from build123d import *

# Parameters (mm, degrees)
F1_DEPTH = 9.8
F2_R     = 1.75
F3_DEPTH = 7
F4_R     = 1.75
F5_DEPTH = 7
F6_W     = 115
F6_H     = 2.2
F7_DEPTH = 7.5
F8_W     = 113.41
F8_H     = 1.6
F9_DEPTH = 233
F10_R    = 2


with BuildPart() as f1:
    # F0 (on Top) → F1 (new body)
    with BuildSketch(Plane.XY):
        Polygon((8.22, 6), (0, 6), (0, 0), (7, 0), (7, -4.8), (125.55, -4.8), (125.55, 0), (132.55, 0), (132.55, 6), (124.33, 6), (124.33, 10), (122.98, 10), (122.98, 6), (9.57, 6), (9.57, 10), (8.22, 10), align=None)
    extrude(amount=F1_DEPTH)

    # F2 (on face) → F3 (cut)
    with BuildSketch(Plane.XZ):
        with Locations((3.5, 4.9)):
            Circle(F2_R)
    extrude(amount=-F3_DEPTH, mode=Mode.SUBTRACT)

    # F4 (on face) → F5 (cut)
    with BuildSketch(Plane.XZ):
        with Locations((129.05, 4.9)):
            Circle(F4_R)
    extrude(amount=-F5_DEPTH, mode=Mode.SUBTRACT)

    # F6 (on face) → F7 (cut)
    with BuildSketch(Plane.XZ.offset(4.8)):
        with Locations((66.275, 4.9)):
            Rectangle(F6_W, F6_H)
    extrude(amount=-F7_DEPTH, mode=Mode.SUBTRACT)

    # F8 (on face) → F9 (join)
    with BuildSketch(Plane(origin=(0, 6, 0), x_dir=(-1, 0, 0), z_dir=(0, 1, 0))):
        with Locations((-66.275, 4.9)):
            Rectangle(F8_W, F8_H)
    extrude(amount=F9_DEPTH)

    # F10
    f10_edges = [f1.edges().sort_by_distance(p)[0] for p in [
        (122.98, 239, 4.9),
        (9.57, 239, 4.9),
    ]]
    fillet(f10_edges, radius=F10_R)


solid = f1.part
Model file for the job. Use its own axes, mm. A direction names the side the tool comes from. Give positions to 0.01 mm unless a question says otherwise; leave off trailing zeros. Loops run counter-clockwise (first coordinate to the right, second up) from the corner with the lowest first, then second, coordinate; pieces in that order, holes last.
1) Wall check: line 1 (Z direction, x = 3.5, y = 3.45); line 2 (Z direction, x = 69, y = 84.5); line 3 (Y direction, x = 124, z = 0.5). Give the ranges that are in metal, low to high.
2) Tool access for faces 4 (the flat face through (7, -2, 5)), 5 (the flat face through (127, 6, 5)), 6 (the flat face through (125.55, -2, 5)): list every direction of +Z, -Z, +X, -X, +Y, -Y with a clear straight run to the whole face (end or side of a thin tool).
3) Saw through at B-B (x = 72). Write the cut outline in (y, z).
4) Saw through at C-C (y = 118). Write the cut outline in (x, z).
5) Saw through at A-A (z = 1.5). Write the cut outline in (x, y).
6) Flat gauge pins, fed straight in: pin 1 Ø1.2 at (y, z) = (7, 2) entering from +X; pin 2 Ø3 at (y, z) = (8.5, 7.5) entering from -X; pin 3 Ø3 at (x, z) = (3.5, 4.9) entering from +Y; pin 4 Ø1 at (x, z) = (32, 2) entering from +Y. Where does each tip first touch, or does it go through?
7) Pull direction Z, two halves, no side cores. Call faces 1 (the flat face through (65, -1, 6)), 2 (the flat face through (132.55, 3, 5)), 3 (the flat face through (65, 1, 0)): +Z half, -Z half, draft (parallel to the pull), parting line (faces both ways), or undercut.
Answer block:
1. line 1: z = 0 to 3.15, 6.65 to 9.8
1. line 2: z = 4.1 to 5.7
1. line 3: y = -4.8 to 10
2. face 4: +Z, -Z, -X, -Y
2. face 5: +Z, -Z, +X, +Y
2. face 6: +Z, -Z, +X, -Y
3. outline: (-4.8, 0) - (6, 0) - (6, 4.1) - (239, 4.1) - (239, 5.7) - (6, 5.7) - (6, 9.8) - (-4.8, 9.8) - (-4.8, 6) - (2.7, 6) - (2.7, 3.8) - (-4.8, 3.8) - close
4. outline: (9.57, 4.1) - (122.98, 4.1) - (122.98, 5.7) - (9.57, 5.7) - close
5. outline: (0, 0) - (7, 0) - (7, -4.8) - (125.55, -4.8) - (125.55, 0) - (132.55, 0) - (132.55, 6) - (124.33, 6) - (124.33, 10) - (122.98, 10) - (122.98, 6) - (9.57, 6) - (9.57, 10) - (8.22, 10) - (8.22, 6) - (0, 6) - close
6. pin 1: stops at x = 124.33
6. pin 2: stops at x = 8.22
6. pin 3: passes through
6. pin 4: stops at y = 6
7. face 1: undercut
7. face 2: draft
7. face 3: -Z half
